Read the model definition and answer for the solid it produces. Units are mm, in the model's axes. A direction names the side the tool comes from. Coordinates: 2 decimals unless noted, no trailing zeros. Order: outer loops, then holes, each group sorted by start corner. A loop starts at its lowest first (then second) coordinate and runs counter-clockwise, first axis right, second up. Notation, with made-up numbers: (-8, 5) -> (42, 5) arc R16 ccw to (42, 34) -> close; hole circle Ø7 at (28.5, 20). An arc over 180 degrees is marked (long way). Answer as a JSON object with one key per item and string values. Group by question number.
1) Section D-D on x = -7.5 is taken. Determine the outline of the cut face in (y, z), and give its area (3 significant figures).
2) Section B-B on y = 1.3 is taken. Determine the outline of the cut face in (x, z), and give its area (3 significant figures).
3) A tool of negligible diameter and unlimited length cuts with its end or side. For faces 1 (the flat face through (0, 2.25, 0.5)), 2 (the flat face through (-2.25, 0, 0.5)), 3 (the flat face through (0, -2.25, 0.5)), 4 (the flat face through (2.25, 0, 0.5)), from which of +Z, -Z, +X, -X, +Y, -Y can it reach the whole face along a straight path? Write none if from no direction.
4) Section C-C on z = -1.6 is taken. Determine the outline of the cut face in (x, y), and give its area (4 significant figures).
5) Given pin 1 (0.8 mm diameter, centred on x = -0.5, z = 0.5, fed in from +Y); pin 2 (0.8 mm diameter, centred on y = 0.5, z = 0.5, fed in from +X); pin 3 (0.8 mm diameter, centred on x = 0.5, z = 0.5, fed in from -Y), each flat-ended and moving along its own axis, determine where each tip first touches the part or whether it passes through.
6) Section A-A on z = 0.55 is taken. Determine the outline of the cut face in (x, y), and give its area (3 significant figures).
7) Consider L1, parallel to Z at x = -8.5, y = 1.15; L2, parallel to X at y = 0.4, z = 0.6. Determine where each line is inside the solid, lowest interval first.
from build123d import *

# Parameters (mm, degrees)
F1_DEPTH = 1
F2_W     = 5
F2_H     = 5
F3_DEPTH = 2


with BuildPart() as f1:
    # F0 (on Top) → F1 (new body)
    with BuildSketch(Plane.XY):
        with BuildLine():
            Line((1.75, 2.25), (-1.75, 2.25))
            ThreePointArc((-1.75, 2.25), (-2.103553, 2.103553), (-2.25, 1.75))
            Line((-2.25, 1.75), (-2.25, -1.75))
            ThreePointArc((-2.25, -1.75), (-2.103553, -2.103553), (-1.75, -2.25))
            Line((-1.75, -2.25), (1.75, -2.25))
            ThreePointArc((1.75, -2.25), (2.103553, -2.103553), (2.25, -1.75))
            Line((2.25, -1.75), (2.25, 1.75))
            ThreePointArc((2.25, 1.75), (2.103553, 2.103553), (1.75, 2.25))
        make_face()
    extrude(amount=F1_DEPTH)

    # F2 (on Top) → F3 (join)
    with BuildSketch(Plane.XY):
        Rectangle(F2_W, F2_H)
        with BuildLine():
            Line((-12.07417, -1.063874), (-2.5, -2.5))
            Line((-2.5, -2.5), (-2.5, 2.5))
            Line((-2.5, 2.5), (-12.07417, 1.063874))
            ThreePointArc((-12.07417, 1.063874), (-12.37887, 0.895684), (-12.5, 0.569406))
            Line((-12.5, 0.569406), (-12.5, -0.569406))
            ThreePointArc((-12.5, -0.569406), (-12.37887, -0.895684), (-12.07417, -1.063874))
        make_face()
        with BuildLine():
            Line((2.5, 2.5), (2.5, -2.5))
            Line((2.5, -2.5), (12.07417, -1.063874))
            ThreePointArc((12.07417, -1.063874), (12.37887, -0.895684), (12.5, -0.569406))
            Line((12.5, -0.569406), (12.5, 0.569406))
            ThreePointArc((12.5, 0.569406), (12.37887, 0.895684), (12.07417, 1.063874))
            Line((12.07417, 1.063874), (2.5, 2.5))
        make_face()
    extrude(amount=-F3_DEPTH)


solid = f1.part
Worked answers:
{
 "1": {"outline": "(-1.75, -2) -> (1.75, -2) -> (1.75, 0) -> (-1.75, 0) -> close", "area": "7.00 mm²"},
 "2": {"outline": "(-10.5, -2) -> (10.5, -2) -> (10.5, 0) -> (2.25, 0) -> (2.25, 1) -> (-2.25, 1) -> (-2.25, 0) -> (-10.5, 0) -> close", "area": "46.5 mm²"},
 "3": {"face 1": "+Z, +X, -X, +Y", "face 2": "+Z, -X, +Y, -Y", "face 3": "+Z, +X, -X, -Y", "face 4": "+Z, +X, +Y, -Y"},
 "4": {"outline": "(-12.5, -0.57) arc R0.5 ccw to (-12.07, -1.06) -> (-2.5, -2.5) -> (2.5, -2.5) -> (12.07, -1.06) arc R0.5 ccw to (12.5, -0.57) -> (12.5, 0.57) arc R0.5 ccw to (12.07, 1.06) -> (2.5, 2.5) -> (-2.5, 2.5) -> (-12.07, 1.06) arc R0.5 ccw to (-12.5, 0.57) -> close", "area": "94.85 mm²"},
 "5": {"pin 1": "stops at y = 2.25", "pin 2": "stops at x = 2.25", "pin 3": "stops at y = -2.25"},
 "6": {"outline": "(-2.25, -1.75) arc R0.5 ccw to (-1.75, -2.25) -> (1.75, -2.25) arc R0.5 ccw to (2.25, -1.75) -> (2.25, 1.75) arc R0.5 ccw to (1.75, 2.25) -> (-1.75, 2.25) arc R0.5 ccw to (-2.25, 1.75) -> close", "area": "20.0 mm²"},
 "7": {"L1": "z = -2 to 0", "L2": "x = -2.25 to 2.25"}
}
